Read the model definition and answer for the solid it produces. Units are mm, in the model's axes. Face numbers are marked on the shaded views. Coordinates: 2 decimals unless noted, no trailing zeros. Write each loop counter-clockwise with the first axis right and the second up, starting at its lowest first coordinate (ties: lowest second). Pieces come first, ordered by that corner, then holes.
(1) The mould has two halves that part along X. Classify the marked faces 1 and 2: +X half, -X half, draft (parallel to the pull), parting line (faces both ways), or undercut.
(2) Given pin 1 (5.5 mm diameter, centred on x = -50, y = -0.5, fed in from -Z); pin 2 (1 mm diameter, centred on x = -7.5, y = 5.5, fed in from +Z), each flat-ended and moving along its own axis, determine where each tip first touches the part or whether it passes through.
(3) Section A-A on z = 4 is taken. Write down the section's boundary in (x, y), then the cut area to 3 significant figures.
(4) Find the intervals of material crossed by probe 1 along X at (y, z) = (0, 2.35); probe 2 along X at (y, z) = (0, 1.3); probe 3 along Y at (x, z) = (50, 0.6), in increasing order.
(5) Section D-D on x = -16.5 is taken. Write down the section's boundary in (y, z).
(6) Section B-B on y = 0 is taken. Write down the section's boundary in (x, z), then the cut area to 3 significant figures.
(7) Section C-C on x = 50 is taken. Write down the section's boundary in (y, z).
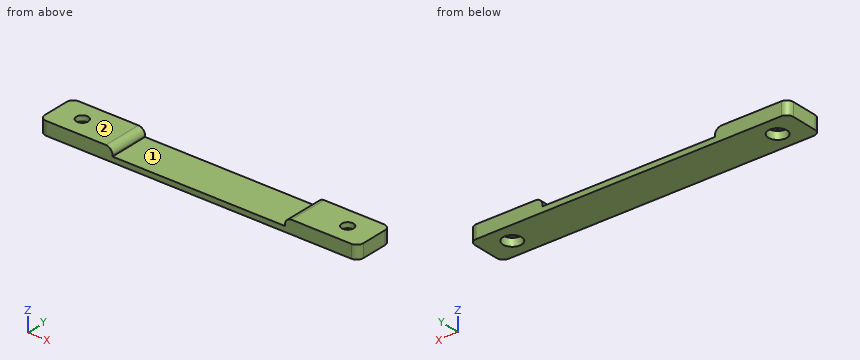
from build123d import *

# Parameters (mm, degrees)
F0_W     = 120
F0_H     = 15
F1_DEPTH = 2
F2_W     = 27.5
F2_H     = 15
F3_DEPTH = 3
F4_R     = 2.25
F5_DEPTH = 5
F6_R     = 2.5
F4_R_2   = 3.5
F7_DEPTH = 3


with BuildPart() as f1:
    # F0 (on Top) → F1 (new body)
    with BuildSketch(Plane.XY):
        Rectangle(F0_W, F0_H)
    extrude(amount=F1_DEPTH)

    # F2 (on face) → F3 (join)
    with BuildSketch(Plane.XY.offset(2)):
        with Locations((-46.25, 0)):
            Rectangle(F2_W, F2_H)
        with Locations((46.25, 0)):
            Rectangle(F2_W, F2_H)
    extrude(amount=F3_DEPTH)

    # F4 (on face) → F5 (cut)
    with BuildSketch(Plane(origin=(0, 0, 0), x_dir=(1, 0, 0), z_dir=(0, 0, -1))):
        with Locations((-50, 0)):
            Circle(F4_R)
        with Locations((50, 0)):
            Circle(F4_R)
    extrude(amount=-F5_DEPTH, mode=Mode.SUBTRACT)

    # F6
    f6_edges = [f1.edges().sort_by_distance(p)[0] for p in [
        (60, 7.5, 2.5),
        (60, -7.5, 2.5),
        (-60, 7.5, 2.5),
        (-60, -7.5, 2.5),
        (32.5, 0, 5),
        (-32.5, 0, 5),
    ]]
    fillet(f6_edges, radius=F6_R)

    # F4 (on face) → F7 (cut)
    with BuildSketch(Plane(origin=(0, 0, 0), x_dir=(1, 0, 0), z_dir=(0, 0, -1))):
        with Locations((-50, 0)):
            Circle(F4_R_2)
        with Locations((-50, 0)):
            Circle(F4_R, mode=Mode.SUBTRACT)
        with Locations((50, 0)):
            Circle(F4_R_2)
        with Locations((50, 0)):
            Circle(F4_R, mode=Mode.SUBTRACT)
    extrude(amount=-F7_DEPTH, mode=Mode.SUBTRACT)


solid = f1.part
Response:
1. face 1: undercut
1. face 2: draft
2. pin 1: stops at z = 3
2. pin 2: stops at z = 2
3. outline: (-60, -5) arc R2.5 ccw to (-57.5, -7.5) - (-33, -7.5) - (-33, 7.5) - (-57.5, 7.5) arc R2.5 ccw to (-60, 5) - close; (33, -7.5) - (57.5, -7.5) arc R2.5 ccw to (60, -5) - (60, 5) arc R2.5 ccw to (57.5, 7.5) - (33, 7.5) - close; hole circle Ø4.5 at (-50, 0); hole circle Ø4.5 at (50, 0)
3. area: 773 mm2
4. probe 1: x = -60 to -53.5, -46.5 to -32.5, 32.5 to 46.5, 53.5 to 60
4. probe 2: x = -60 to -53.5, -46.5 to 46.5, 53.5 to 60
4. probe 3: y = -7.5 to -3.5, 3.5 to 7.5
5. outline: (-7.5, 0) - (7.5, 0) - (7.5, 2) - (-7.5, 2) - close
6. outline: (-60, 0) - (-53.5, 0) - (-53.5, 3) - (-52.25, 3) - (-52.25, 5) - (-60, 5) - close; (-47.75, 3) - (-46.5, 3) - (-46.5, 0) - (46.5, 0) - (46.5, 3) - (47.75, 3) - (47.75, 5) - (35, 5) arc R2.5 ccw to (32.5, 2.5) - (32.5, 2) - (-32.5, 2) - (-32.5, 2.5) arc R2.5 ccw to (-35, 5) - (-47.75, 5) - close; (52.25, 3) - (53.5, 3) - (53.5, 0) - (60, 0) - (60, 5) - (52.25, 5) - close
6. area: 342 mm2
7. outline: (-7.5, 0) - (-3.5, 0) - (-3.5, 3) - (-2.25, 3) - (-2.25, 5) - (-7.5, 5) - close; (2.25, 3) - (3.5, 3) - (3.5, 0) - (7.5, 0) - (7.5, 5) - (2.25, 5) - close
